Design review of the part built by this model. Coordinates are the model's own, in mm. Face numbers are marked on the shaded views. A direction names the side the tool comes from. Coordinates: 2 decimals unless noted, no trailing zeros. Loops run counter-clockwise (first coordinate to the right, second up) from the corner with the lowest first, then second, coordinate; pieces in that order, holes last. Notation, with made-up numbers: M -23,33.5 L 13,33.5 A22 cw 13,56.5 Z; hole C 6.5,83 d8. An arc over 180 degrees is marked long. Write item = value, one per line. Start each with the question number.
```python
from build123d import *

# Parameters (mm, degrees)
F0_R     = 63.5
F0_R_2   = 6.35
F0_W     = 12.7
F0_H     = 50.8
F0_W_2   = 25.4
F1_DEPTH = 12.7
F2_DEPTH = 63.5
F3_DEPTH = 12.7
F5_DEPTH = 88.901
F4_R     = 9.525
F6_DEPTH = 88.901
F7_R     = 3.81


with BuildPart() as f1:
    # F0 (on Top) → F1 (new body)
    with BuildSketch(Plane.XY):
        Circle(F0_R)
        with Locations((0, -44.45)):
            Circle(F0_R_2, mode=Mode.SUBTRACT)
        with Locations((-44.45, 0)):
            Circle(F0_R_2, mode=Mode.SUBTRACT)
        Polygon((-25.4, -25.4), (-25.4, 25.4), (-12.7, 25.4), (12.7, 25.4), (25.4, 25.4), (25.4, -25.4), (12.7, -25.4), (-12.7, -25.4), align=None, mode=Mode.SUBTRACT)
        with Locations((44.45, 0)):
            Circle(F0_R_2, mode=Mode.SUBTRACT)
        with Locations((0, 44.45)):
            Circle(F0_R_2, mode=Mode.SUBTRACT)
        with Locations((-19.05, 0)):
            Rectangle(F0_W, F0_H)
        Rectangle(F0_W_2, F0_H)
        with Locations((19.05, 0)):
            Rectangle(F0_W, F0_H)
    extrude(amount=-F1_DEPTH)

    # F0 (on Top) → F2 (join)
    with BuildSketch(Plane.XY):
        with Locations((-19.05, 0)):
            Rectangle(F0_W, F0_H)
        with Locations((19.05, 0)):
            Rectangle(F0_W, F0_H)
    extrude(amount=F2_DEPTH)

    # F0 (on Top) → F3 (join)
    with BuildSketch(Plane.XY):
        Rectangle(F0_W_2, F0_H)
    extrude(amount=F3_DEPTH)

    # F4 (on face) → F5 (cut, through all)
    with BuildSketch(Plane.YZ.offset(25.4)):
        with BuildLine():
            Line((-25.4, 63.5), (-25.4, 38.1))
            ThreePointArc((-25.4, 38.1), (-17.960512, 56.060512), (0, 63.5))
            Line((0, 63.5), (-25.4, 63.5))
        make_face()
        with BuildLine():
            ThreePointArc((0, 63.5), (17.960512, 56.060512), (25.4, 38.1))
            Line((25.4, 38.1), (25.4, 63.5))
            Line((25.4, 63.5), (0, 63.5))
        make_face()
    extrude(amount=-F5_DEPTH, mode=Mode.SUBTRACT)

    # F4 (on face) → F6 (cut, through all)
    with BuildSketch(Plane.YZ.offset(25.4)):
        with Locations((0, 38.1)):
            Circle(F4_R)
    extrude(amount=-F6_DEPTH, mode=Mode.SUBTRACT)

    # F7
    f7_edges = [f1.edges().sort_by_distance(p)[0] for p in [
        (25.4, 0, 0),
        (0, -25.4, 0),
        (-25.4, 0, 0),
        (0, 25.4, 0),
        (-63.5, 0, 0),
    ]]
    fillet(f7_edges, radius=F7_R)


solid = f1.part
```
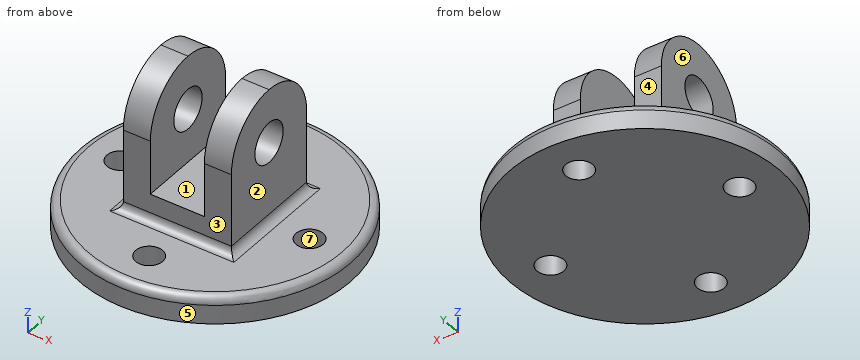
(1) To check wall thickness, follow L1, parallel to Y at x = 0, z = -5; L2, parallel to Y at x = -21, z = 38; L3, parallel to X at y = 15.5, z = 21.5. State the ranges of each line that lie inside material, in increasing order.
(2) Tool access review of the marked faces 1, 2, 3 and 4: name each direction out of +Z, -Z, +X, -X, +Y, -Y from which nothing blocks a thin tool from reaching the whole face with its end or side.
(3) Mouldability with a two-part tool opening along X and no side actions: class the marked faces 5, 6 and 7 as +X half, -X half, draft (parallel to the pull), parting line (faces both ways), or undercut.
(4) Take a section at C-C (x = 2). Give the number of separate pieces and of enclosed holes in the cut face, plus the area to 3 significant figures.
(5) Insertion check: pin 1 (2 mm diameter, centred on y = 11, z = 37, fed in from -X); pin 2 (12 mm diameter, centred on x = 10, z = 18.5, fed in from +Y); pin 3 (20.5 mm diameter, centred on x = 44.45, y = 0, fed in from +Z); pin 4 (7.5 mm diameter, centred on x = 0, y = 44.45, fed in from +Z). Each pin has a flat end and moves straight along its axis. Give the tip position at first contact, or say it passes through.
(6) Take a section at A-A (z = 41.5). State the section outline as (x, y) points, plus the area to 3 significant figures.
(7) Take a section at B-B (z = 57). State the section outline as (x, y) points.
Results list:
q1.L1 = -63.5 to -50.8, -38.1 to 38.1, 50.8 to 63.5
q1.L2 = -25.4 to -9.52, 9.52 to 25.4
q1.L3 = -25.4 to -12.7, 12.7 to 25.4
q2.face_1 = +Z, +Y, -Y
q2.face_2 = +Z, +X, +Y, -Y
q2.face_3 = +Z, +X, -X, -Y
q2.face_4 = +Z, +X, -X, +Y
q3.face_5 = parting line
q3.face_6 = -X half
q3.face_7 = undercut
q4.separate_pieces = 3
q4.enclosed_holes = 0
q4.area = 1,950 mm^2
q5.pin_1 = -25.4
q5.pin_2 = 25.4
q5.pin_3 = 0
q5.pin_4 = through
q6.outline = M -25.4,-25.17 L -12.7,-25.17 L -12.7,-8.9 L -25.4,-8.9 Z; M -25.4,8.9 L -12.7,8.9 L -12.7,25.17 L -25.4,25.17 Z; M 12.7,-25.17 L 25.4,-25.17 L 25.4,-8.9 L 12.7,-8.9 Z; M 12.7,8.9 L 25.4,8.9 L 25.4,25.17 L 12.7,25.17 Z
q6.area = 827 mm^2
q7.outline = M -25.4,-16.97 L -12.7,-16.97 L -12.7,16.97 L -25.4,16.97 Z; M 12.7,-16.97 L 25.4,-16.97 L 25.4,16.97 L 12.7,16.97 Z
